Model file for the job. Use its own axes, mm. Face numbers are marked on the shaded views. A direction names the side the tool comes from. Give positions to 0.01 mm unless a question says otherwise; leave off trailing zeros. Order: outer loops, then holes, each group sorted by start corner. A loop starts at its lowest first (then second) coordinate and runs counter-clockwise, first axis right, second up. Notation, with made-up numbers: (8, 56.5) - (15, 56.5) arc R18 ccw to (15, 74.5) - close; hole circle Ø5 at (-12.5, 48). An arc over 180 degrees is marked (long way). Use CSV: the item, a comma, the result in double quotes. Start each with the question number.
(1) Band-saw the part on A-A, the plane z = 3.2. Give the cut face in (x, y), then the cut area to 3 significant figures.
(2) Probe L1, parallel to Y at x = -8.25, z = 1.9; L2, parallel to Y at x = -7.75, z = 1.55; L3, parallel to Y at x = -14.5, z = 1.8. List the from-to ranges inside material, lowest first.
(3) Drop flat-ended pins along their axis: pin 1 Ø2 at (y, z) = (-28, 3.5) entering from +X; pin 2 Ø2.5 at (x, z) = (-14.5, 2) entering from -Y; pin 3 Ø3 at (x, z) = (-6.5, 3.5) entering from -Y. Give the stop position or say it passes through.
(4) Pull direction Y, two halves, no side cores. Call the marked faces 1, 2 and 3: +Y half, -Y half, draft (parallel to the pull), parting line (faces both ways), or undercut.
(5) Tool access for the marked faces 4, 5 and 6: list every direction of +Z, -Z, +X, -X, +Y, -Y with a clear straight run to the whole face (end or side of a thin tool).
(6) Band-saw the part on C-C, the plane x = -1.25. Give the cut face in (y, z).
(7) Band-saw the part on B-B, the plane y = -19. Give the cut face in (x, z).
from build123d import *

# Parameters (mm, degrees)
ESQUISSE1_R             = 1
ESQUISSE1_R_2           = 1.5
BOSS_EXTRU_1_DEPTH      = 5
ENL_V_MAT_EXTRU_1_DEPTH = 5
ESQUISSE3_W             = 20
ESQUISSE3_H             = 34
BOSS_EXTRU_2_DEPTH      = 5
ESQUISSE4_R             = 1.5
ESQUISSE4_W             = 9.798464728
ESQUISSE4_H             = 39.858161606
ENL_V_MAT_EXTRU_2_DEPTH = 5
ESQUISSE5_W             = 2.5
ESQUISSE5_H             = 34
BOSS_EXTRU_3_DEPTH      = 5
ESQUISSE6_R             = 1.6
BOSS_EXTRU_4_DEPTH      = 5
CONG_1_R                = 10
ESQUISSE7_W             = 40.251504125
ESQUISSE7_H             = 45.079075122
ENL_V_MAT_EXTRU_3_DEPTH = 10
ESQUISSE8_W             = 20
ESQUISSE8_H             = 39.5
ESQUISSE8_R             = 1.5
BOSS_EXTRU_5_DEPTH      = 5
ESQUISSE9_R             = 1.6
BOSS_EXTRU_6_DEPTH      = 5
ESQUISSE10_R            = 1.5
ENL_V_MAT_EXTRU_4_DEPTH = 10
ESQUISSE11_R            = 1.5
ENL_V_MAT_EXTRU_5_DEPTH = 10
BOSS_EXTRU_7_DEPTH      = 5


with BuildPart() as part:
    # Esquisse1 → Boss.-Extru.1 (new body)
    with BuildSketch(Plane.XY):
        with BuildLine():
            Line((-13.584596858, -30.047129187), (-13.584596858, -25.547129187))
            Line((-13.584596858, -25.547129187), (-13.584596858, -25.297129187))
            Line((-13.584596858, -25.297129187), (-13.834596858, -25.297129187))
            Line((-13.834596858, -25.297129187), (-16.334596858, -25.297129187))
            Line((-16.334596858, -25.297129187), (-16.584596858, -25.297129187))
            Line((-16.584596858, -25.297129187), (-16.584596858, -25.047129187))
            Line((-16.584596858, -25.047129187), (-16.584596858, 6.452870813))
            Line((-16.584596858, 6.452870813), (-16.584596858, 6.702870813))
            Line((-16.584596858, 6.702870813), (-16.334596858, 6.702870813))
            Line((-16.334596858, 6.702870813), (-13.834596858, 6.702870813))
            Line((-13.834596858, 6.702870813), (-13.584596858, 6.702870813))
            Line((-13.584596858, 6.702870813), (-13.584596858, 6.952870813))
            Line((-13.584596858, 6.952870813), (-13.584596858, 11.452870813))
            Line((-13.584596858, 11.452870813), (-13.584596858, 11.702870813))
            Line((-13.584596858, 11.702870813), (-13.334596858, 11.702870813))
            Line((-13.334596858, 11.702870813), (-8.584596858, 11.702870813))
            Line((-8.584596858, 11.702870813), (-8.584596858, 6.702870813))
            Line((-8.584596858, 6.702870813), (-7.491776281, 6.702870813))
            Line((-7.491776281, 6.702870813), (-4.034541178, 6.702870813))
            ThreePointArc((-4.034541178, 6.702870813), (-0.161557832, 6.19424756), (3.448773595, 4.702870813))
            ThreePointArc((3.448773595, 4.702870813), (10.66943645, 1.720117321), (18.415403142, 0.702870813))
            ThreePointArc((18.415403142, 0.702870813), (28.415403142, -9.297129187), (18.415403142, -19.297129187))
            ThreePointArc((18.415403142, -19.297129187), (10.66943645, -20.314375694), (3.448773595, -23.297129187))
            ThreePointArc((3.448773595, -23.297129187), (-0.161557832, -24.788505933), (-4.034541178, -25.297129187))
            Line((-4.034541178, -25.297129187), (-7.491776281, -25.297129187))
            Line((-7.491776281, -25.297129187), (-8.584596858, -25.297129187))
            Line((-8.584596858, -25.297129187), (-8.584596858, -30.297129187))
            Line((-8.584596858, -30.297129187), (-13.334596858, -30.297129187))
            Line((-13.334596858, -30.297129187), (-13.584596858, -30.297129187))
            Line((-13.584596858, -30.297129187), (-13.584596858, -30.047129187))
        make_face()
        with Locations((18.477857718, -2.297129187)):
            Circle(ESQUISSE1_R, mode=Mode.SUBTRACT)
        with Locations((25.415403142, -9.359583762)):
            Circle(ESQUISSE1_R, mode=Mode.SUBTRACT)
        with Locations((18.415403142, -9.297129187)):
            Circle(ESQUISSE1_R_2, mode=Mode.SUBTRACT)
        with Locations((11.415403142, -9.234674611)):
            Circle(ESQUISSE1_R, mode=Mode.SUBTRACT)
        with Locations((18.352948567, -16.297129187)):
            Circle(ESQUISSE1_R, mode=Mode.SUBTRACT)
    extrude(amount=BOSS_EXTRU_1_DEPTH)

    # Esquisse2 → Enlèv. mat.-Extru.1 (cut)
    with BuildSketch(Plane(origin=(0, 0, 0), x_dir=(-1, 0, 0), z_dir=(0, 0, -1))):
        Polygon((1.584596858, -19.297129187), (1.584596858, -25.297129187), (1.584596858, -26.297129187), (21.584596858, -26.297129187), (21.584596858, -33.65697819), (-26.833247513, -33.65697819), (-26.198667142, -19.297129187), align=None)
        Polygon((21.584596858, 7.702870813), (1.584596858, 7.702870813), (1.584596858, 6.702870813), (1.584596858, 0.702870813), (-26.198667142, 0.702870813), (-26.833247513, 15.062719816), (21.584596858, 15.062719816), align=None)
    extrude(amount=-ENL_V_MAT_EXTRU_1_DEPTH, mode=Mode.SUBTRACT)

    # Esquisse3 → Boss.-Extru.2 (add)
    with BuildSketch(Plane(origin=(0, 0, 0), x_dir=(-1, 0, 0), z_dir=(0, 0, -1))):
        with Locations((11.584596858, -9.297129187)):
            Rectangle(ESQUISSE3_W, ESQUISSE3_H)
    extrude(amount=-BOSS_EXTRU_2_DEPTH)

    # Esquisse4 → Enlèv. mat.-Extru.2 (cut)
    with BuildSketch(Plane(origin=(0, 0, 0), x_dir=(-1, 0, 0), z_dir=(0, 0, -1))):
        with Locations((9.084596858, -22.797129187)):
            Circle(ESQUISSE4_R)
        with Locations((9.084596858, 4.202870813)):
            Circle(ESQUISSE4_R)
        with Locations((23.983829222, -9.020336398)):
            Rectangle(ESQUISSE4_W, ESQUISSE4_H)
    extrude(amount=-ENL_V_MAT_EXTRU_2_DEPTH, mode=Mode.SUBTRACT)

    # Esquisse5 → Boss.-Extru.3 (add)
    with BuildSketch(Plane(origin=(0, 0, 0), x_dir=(-1, 0, 0), z_dir=(0, 0, -1))):
        with Locations((0.334596858, -9.297129187)):
            Rectangle(ESQUISSE5_W, ESQUISSE5_H)
    extrude(amount=-BOSS_EXTRU_3_DEPTH)

    # Esquisse6 → Boss.-Extru.4 (add)
    # profile 1 of 2: a face of its own
    with BuildSketch(Plane(origin=(0, 0, 0), x_dir=(-1, 0, 0), z_dir=(0, 0, -1))):
        with BuildLine():
            Line((12.324596858, -25.12480516), (5.844596858, -25.12480516))
            Line((5.844596858, -25.12480516), (5.844596858, -28.797129187))
            ThreePointArc((5.844596858, -28.797129187), (9.084596858, -32.037129187), (12.324596858, -28.797129187))
            Line((12.324596858, -28.797129187), (12.324596858, -25.12480516))
        make_face()
        with Locations((9.084596858, -28.797129187)):
            Circle(ESQUISSE6_R, mode=Mode.SUBTRACT)
    # profile 2 of 2: a face of its own
    with BuildSketch(Plane(origin=(0, 0, 0), x_dir=(-1, 0, 0), z_dir=(0, 0, -1))):
        with BuildLine():
            Line((12.324596858, 6.757738308), (5.844596858, 6.757738308))
            Line((5.844596858, 6.757738308), (5.844596858, 10.202870813))
            ThreePointArc((5.844596858, 10.202870813), (9.084596858, 13.442870813), (12.324596858, 10.202870813))
            Line((12.324596858, 10.202870813), (12.324596858, 6.757738308))
        make_face()
        with Locations((9.084596858, 10.202870813)):
            Circle(ESQUISSE6_R, mode=Mode.SUBTRACT)
    extrude(amount=-BOSS_EXTRU_4_DEPTH)

    # Congé1
    # the kernel refuses this fillet: 10 mm, written as the material it adds along each edge
    with BuildSketch(Plane(origin=(0.915403142, 0.702870813, 0), x_dir=(1, 0, 0), z_dir=(0, 0, 1))) as cong_1_piece_1:
        with BuildLine():
            CenterArc((9.539392014, 10), CONG_1_R, 197.457603124, 72.542396876)
            Line((0, 7), (-0.19078784, 6.94))
            ThreePointArc((-0.19078784, 6.94), (-0.2, 3.5), (-0.2, 0))
            Line((-0.2, 0), (0, -0.2))
            Line((0, -0.2), (9.539392014, -0.2))
            Line((9.539392014, -0.2), (9.539392014, 0))
        make_face()
    extrude(amount=5)
    with BuildSketch(Plane(origin=(0.915403142, -19.297129187, 5), x_dir=(0, -1, 0), z_dir=(0, 0, -1))) as cong_1_piece_2:
        with BuildLine():
            CenterArc((10, -9.539392014), CONG_1_R, 107.457603124, 72.542396876)
            Line((0, -9.539392014), (-0.2, -9.539392014))
            Line((-0.2, -9.539392014), (-0.2, 0))
            Line((-0.2, 0), (0, 0.2))
            ThreePointArc((0, 0.2), (3.5, 0.2), (6.94, 0.19078784))
            Line((6.94, 0.19078784), (7, 0))
        make_face()
    extrude(amount=5)

    # Esquisse7 → Enlèv. mat.-Extru.3 (cut)
    with BuildSketch(Plane(origin=(0, 0, 0), x_dir=(-1, 0, 0), z_dir=(0, 0, -1))):
        with Locations((-21.041155205, -11.091158949)):
            Rectangle(ESQUISSE7_W, ESQUISSE7_H)
    extrude(amount=-ENL_V_MAT_EXTRU_3_DEPTH, mode=Mode.SUBTRACT)

    # Esquisse8 → Boss.-Extru.5 (add)
    with BuildSketch(Plane(origin=(0, 0, 0), x_dir=(-1, 0, 0), z_dir=(0, 0, -1))):
        with Locations((9.084596858, -6.547129187)):
            Rectangle(ESQUISSE8_W, ESQUISSE8_H)
        with Locations((9.084596858, -22.797129187)):
            Circle(ESQUISSE8_R, mode=Mode.SUBTRACT)
    extrude(amount=-BOSS_EXTRU_5_DEPTH)

    # Esquisse9 → Boss.-Extru.6 (add)
    with BuildSketch(Plane(origin=(0, 0, 0), x_dir=(-1, 0, 0), z_dir=(0, 0, -1))):
        with BuildLine():
            Line((12.324596858, 15.702870813), (12.324596858, 13.202870813))
            Line((12.324596858, 13.202870813), (10.308361541, 13.202870813))
            ThreePointArc((10.308361541, 13.202870813), (9.084596858, 13.442870813), (7.860832174, 13.202870813))
            Line((7.860832174, 13.202870813), (5.844596858, 13.202870813))
            Line((5.844596858, 13.202870813), (5.844596858, 15.702870813))
            ThreePointArc((5.844596858, 15.702870813), (9.084596858, 18.942870813), (12.324596858, 15.702870813))
        make_face()
        with Locations(Location((9.084596858, 15.702870813, 0), (0, 0, 180))):
            Circle(ESQUISSE9_R, mode=Mode.SUBTRACT)
    extrude(amount=-BOSS_EXTRU_6_DEPTH)

    # Esquisse10 → Enlèv. mat.-Extru.4 (cut)
    with BuildSketch(Plane(origin=(0, 0, 0), x_dir=(-1, 0, 0), z_dir=(0, 0, -1))):
        with Locations(Location((9.084596858, 9.702870813, 0), (0, 0, 180))):
            Circle(ESQUISSE10_R)
    extrude(amount=-ENL_V_MAT_EXTRU_4_DEPTH, mode=Mode.SUBTRACT)

    # Esquisse11 → Enlèv. mat.-Extru.5 (cut)
    with BuildSketch(Plane(origin=(0, 0, 0), x_dir=(-1, 0, 0), z_dir=(0, 0, -1))):
        with Locations((9.084596858, -20.047129187)):
            Circle(ESQUISSE11_R)
        with Locations((9.084596858, 6.952870813)):
            Circle(ESQUISSE11_R)
    extrude(amount=-ENL_V_MAT_EXTRU_5_DEPTH, mode=Mode.SUBTRACT)

    # Esquisse12 → Boss.-Extru.7 (add)
    with BuildSketch(Plane(origin=(0, 0, 0), x_dir=(-1, 0, 0), z_dir=(0, 0, -1))):
        with BuildLine():
            ThreePointArc((9.684075798, 8.327870813), (9.084596858, 11.202870813), (8.485117917, 8.327870813))
            ThreePointArc((8.485117917, 8.327870813), (9.084596858, 8.452870813), (9.684075798, 8.327870813))
        make_face()
        with BuildLine():
            ThreePointArc((8.485117917, -21.422129187), (9.084596858, -24.297129187), (9.684075798, -21.422129187))
            ThreePointArc((9.684075798, -21.422129187), (9.084596858, -21.547129187), (8.485117917, -21.422129187))
        make_face()
    extrude(amount=-BOSS_EXTRU_7_DEPTH)


solid = part.part
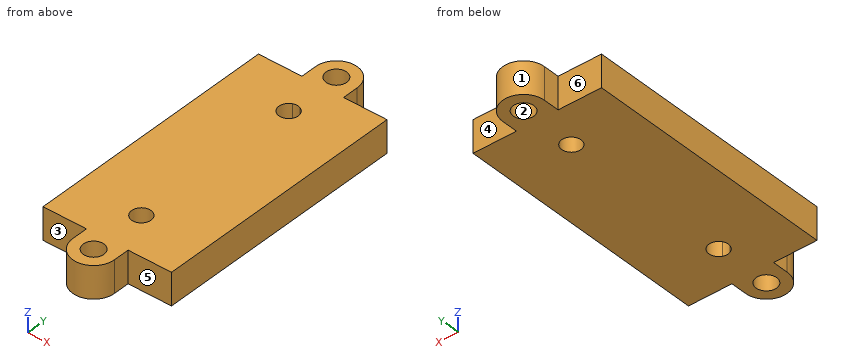
Answer block:
1,outline,"(-19.08, -26.3) - (-12.32, -26.3) - (-12.32, -28.8) arc R3.24 ccw to (-5.84, -28.8) - (-5.84, -26.3) - (0.92, -26.3) - (0.92, 13.2) - (-5.84, 13.2) - (-5.84, 15.7) arc R3.24 ccw to (-12.32, 15.7) - (-12.32, 13.2) - (-19.08, 13.2) - close; hole circle Ø3.2 at (-9.08, -28.8); hole circle Ø3.2 at (-9.08, 15.7); hole circle Ø3 at (-9.08, -20.05); hole circle Ø3 at (-9.08, 6.95)"
1,area,"825 mm2"
2,L1,"y = -31.93 to -30.16, -27.43 to -21.29, -18.8 to 5.71, 8.2 to 14.34, 17.07 to 18.83"
2,L2,"y = -31.75 to -29.68, -27.91 to -20.73, -19.36 to 6.27, 7.64 to 14.82, 16.59 to 18.66"
2,L3,"y = -26.3 to 13.2"
3,pin 1,"stops at x = -5.84"
3,pin 2,"stops at y = -26.3"
3,pin 3,"stops at y = -31.85"
4,face 1,"+Y half"
4,face 2,"undercut"
4,face 3,"-Y half"
5,face 4,"+Z, -Z, +X, +Y"
5,face 5,"+Z, -Z, +X, -Y"
5,face 6,"+Z, -Z, -X, +Y"
6,outline,"(-26.3, 0) - (13.2, 0) - (13.2, 5) - (-26.3, 5) - close"
7,outline,"(-19.08, 0) - (-10.16, 0) - (-10.16, 5) - (-19.08, 5) - close; (-8.01, 0) - (0.92, 0) - (0.92, 5) - (-8.01, 5) - close"
